Part print with two shaded views. Sizes in mm from the minimum x, y, z corner. Coordinates: 2 decimals unless noted, no trailing zeros. Loops run counter-clockwise (first coordinate to the right, second up) from the corner with the lowest first, then second, coordinate; pieces in that order, holes last. Notation, with made-up numbers: (8, 65) -> (55, 65) arc R24 cw to (55, 80) -> close; hole circle Ø10 at (29.25, 36). An arc over 180 degrees is marked (long way). Write each question's results on one line, items separated by ' | '.
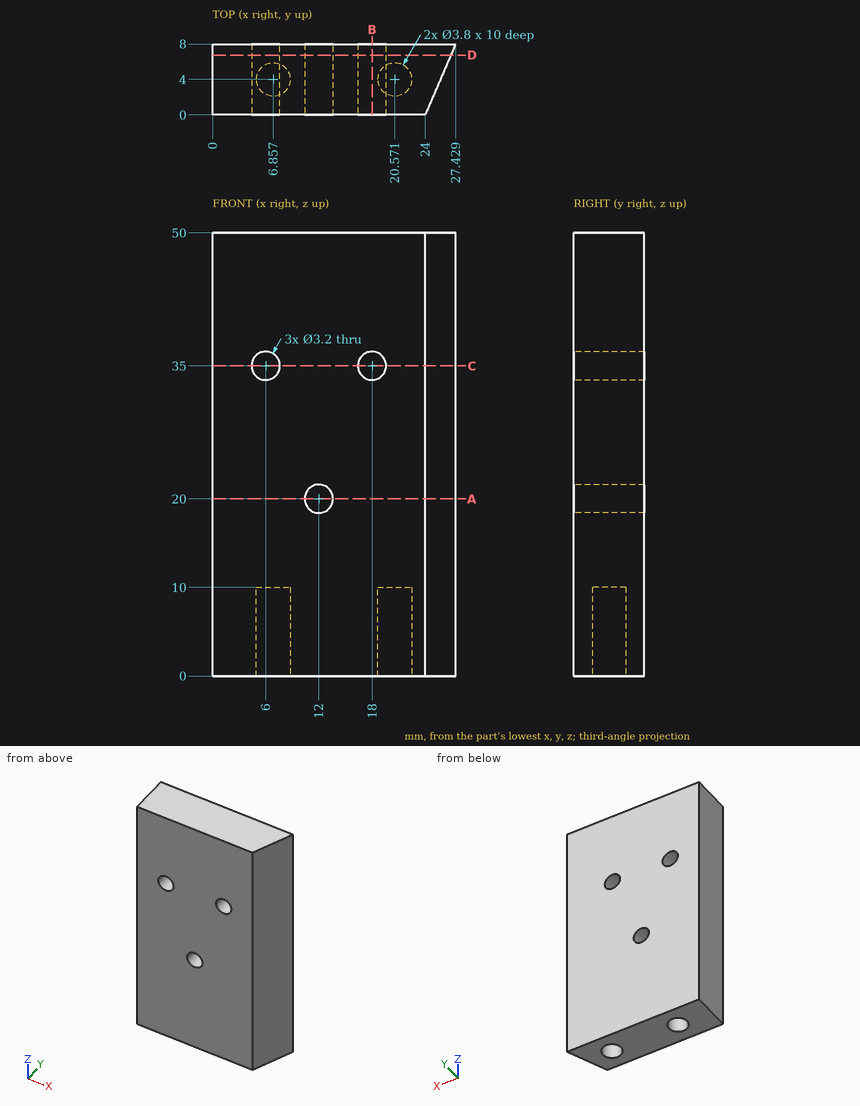
Q1. Drop flat-ended pins along their axis: pin 1 (3 mm diameter, centred on y = 1, z = 9, fed in from +X); pin 2 (1.9 mm diameter, centred on x = 7.5, y = 4, fed in from -Z); pin 3 (2 mm diameter, centred on y = 3, z = 33.5, fed in from +X) (1 decimal); pin 4 (2.5 mm diameter, centred on x = 6, z = 35, fed in from +Y). Give the stop position or say it passes through.
Results are:
pin 1: x = 25.07 | pin 2: z = 10 | pin 3: x = 25.7 | pin 4: through
Q2. Cut at D-D on y = 6.75. Write the cut outline in (x, z).
Results are:
outline: (0, 0) -> (26.89, 0) -> (26.89, 50) -> (0, 50) -> close; hole circle Ø3.2 at (6, 35); hole circle Ø3.2 at (12, 20); hole circle Ø3.2 at (18, 35)
Q3. Cut at A-A on z = 20. Write the cut outline in (x, y).
Results are:
outline: (0, 0) -> (10.4, 0) -> (10.4, 8) -> (0, 8) -> close; (13.6, 0) -> (24, 0) -> (27.43, 8) -> (13.6, 8) -> close
Q4. Cut at B-B on x = 18. Write the cut outline in (y, z).
Results are:
outline: (0, 0) -> (8, 0) -> (8, 33.4) -> (0, 33.4) -> close; (0, 36.6) -> (8, 36.6) -> (8, 50) -> (0, 50) -> close
Q5. Wall check: L1, parallel to X at y = 4, z = 7.25 (1 decimal); L2, parallel to Z at x = 4.75, y = 4.5; L3, parallel to Z at x = 12.75, y = 3.5 (1 decimal). Give the ranges that are in metal, low to high. Write a range as from..to.
Results are:
L1: 0..5, 8.8..18.7, 22.5..25.7 | L2: 0..34, 36..50 | L3: 0..18.6, 21.4..50
Q6. Cut at C-C on z = 35. Write the cut outline in (x, y).
Results are:
outline: (0, 0) -> (4.4, 0) -> (4.4, 8) -> (0, 8) -> close; (7.6, 0) -> (16.4, 0) -> (16.4, 8) -> (7.6, 8) -> close; (19.6, 0) -> (24, 0) -> (27.43, 8) -> (19.6, 8) -> close
